```python
from build123d import *

# Parameters (mm, degrees)
F0_W     = 177.8
F0_H     = 101.6
F0_W_2   = 38.1
F0_H_2   = 38.1
F1_DEPTH = 25.4
F2_DEPTH = 0.254


with BuildPart() as f1:
    # F0 (on Front) → F1 (new body)
    with BuildSketch(Plane.XZ):
        with Locations((6.545865, 10.16)):
            Rectangle(F0_W, F0_H)
        with Locations((-62.417315, -15.311638)):
            Rectangle(F0_W_2, F0_H_2, mode=Mode.SUBTRACT)
        with Locations((7.015266, -19.05)):
            Rectangle(F0_W_2, F0_H_2, mode=Mode.SUBTRACT)
        with Locations((66.230962, -19.05)):
            Rectangle(F0_W_2, F0_H_2, mode=Mode.SUBTRACT)
        with Locations((-62.417315, 38.729876)):
            Rectangle(F0_W_2, F0_H_2, mode=Mode.SUBTRACT)
        with Locations((63.931333, 33.843145)):
            Rectangle(F0_W_2, F0_H_2, mode=Mode.SUBTRACT)
        with Locations((7.015266, 38.729876)):
            Rectangle(F0_W_2, F0_H_2, mode=Mode.SUBTRACT)
    extrude(amount=F1_DEPTH)

    # F0 (on Front) → F2 (join)
    with BuildSketch(Plane.XZ):
        with Locations((-62.417315, 38.729876)):
            Rectangle(F0_W_2, F0_H_2)
        with Locations((7.015266, 38.729876)):
            Rectangle(F0_W_2, F0_H_2)
        with Locations((63.931333, 33.843145)):
            Rectangle(F0_W_2, F0_H_2)
        with Locations((66.230962, -19.05)):
            Rectangle(F0_W_2, F0_H_2)
        with Locations((7.015266, -19.05)):
            Rectangle(F0_W_2, F0_H_2)
        with Locations((-62.417315, -15.311638)):
            Rectangle(F0_W_2, F0_H_2)
    extrude(amount=F2_DEPTH)


solid = f1.part
```
Design review of the part built by this model. Coordinates are the model's own, in mm. A direction names the side the tool comes from. Give positions to 0.01 mm unless a question says otherwise; leave off trailing zeros. Order: outer loops, then holes, each group sorted by start corner. A loop starts at its lowest first (then second) coordinate and runs counter-clockwise, first axis right, second up. Notation, with made-up numbers: (83.25, 53.25) -> (132.25, 53.25) arc R14 cw to (132.25, 60.25) -> close; hole circle Ø7 at (-15.5, 38). An arc over 180 degrees is marked (long way). Write each question's results on one line, items separated by ' | '. Start each with the question number.
Q1. Wall thickness on L1, parallel to X at y = -18.25, z = 50.5; L2, parallel to Z at x = -60.5, y = -1.25; L3, parallel to X at y = -0.75, z = -15.5: over which ranges is each line inside the solid? List them lowest first. Write a range as from..to.
Q2. Add section A-A on x = -67.5. Give the boundary of the cut face in (y, z).
Q3. Mouldability with a two-part tool opening along Z and no side actions: class faces 1 (the flat face through (5, -25.4, 11)), 2 (the flat face through (7, -13, -38.1)) as +Z half, -Z half, draft (parallel to the pull), parting line (faces both ways), or undercut.
Q4. Add section B-B on y = -4. Give the boundary of the cut face in (x, z), and give its area (3 significant figures).
Q5. Add section C-C on z = -31. Give the boundary of the cut face in (x, y).
Q6. Machinability: for faces 3 (the flat face through (-43.367, -13, 38)), 4 (the flat face through (95.446, -13, 9)), which of the approach directions +Z, -Z, +X, -X, +Y, -Y give a long, thin tool a straight path to every point of the face, cutting with its end or side? Answer none if there is none.
Q7. For pin 1 (8 mm diameter, centred on x = 6.5, z = -28, fed in from -Y), flat-tipped, find the tip position at first contact; note if it passes through.
Found:
1) L1: x = -82.35..-81.47, -43.37..-12.03, 26.07..44.88, 82.98..95.45 | L2: z = -40.64..-34.36, 3.74..19.68, 57.78..60.96 | L3: x = -82.35..-81.47, -43.37..-12.03, 26.07..47.18, 85.28..95.45
2) outline: (-25.4, -40.64) -> (0, -40.64) -> (0, 60.96) -> (-25.4, 60.96) -> (-25.4, 57.78) -> (-0.25, 57.78) -> (-0.25, 19.68) -> (-25.4, 19.68) -> (-25.4, 3.74) -> (-0.25, 3.74) -> (-0.25, -34.36) -> (-25.4, -34.36) -> close
3) face 1: draft | face 2: undercut
4) outline: (-82.35, -40.64) -> (95.45, -40.64) -> (95.45, 60.96) -> (-82.35, 60.96) -> close; hole (-81.47, -34.36) -> (-43.37, -34.36) -> (-43.37, 3.74) -> (-81.47, 3.74) -> close; hole (-81.47, 19.68) -> (-43.37, 19.68) -> (-43.37, 57.78) -> (-81.47, 57.78) -> close; hole (-12.03, -38.1) -> (26.07, -38.1) -> (26.07, 0) -> (-12.03, 0) -> close; hole (-12.03, 19.68) -> (26.07, 19.68) -> (26.07, 57.78) -> (-12.03, 57.78) -> close; hole (44.88, 14.79) -> (82.98, 14.79) -> (82.98, 52.89) -> (44.88, 52.89) -> close; hole (47.18, -38.1) -> (85.28, -38.1) -> (85.28, 0) -> (47.18, 0) -> close | area: 9,350 mm2
5) outline: (-82.35, -25.4) -> (-81.47, -25.4) -> (-81.47, -0.25) -> (-43.37, -0.25) -> (-43.37, -25.4) -> (-12.03, -25.4) -> (-12.03, -0.25) -> (26.07, -0.25) -> (26.07, -25.4) -> (47.18, -25.4) -> (47.18, -0.25) -> (85.28, -0.25) -> (85.28, -25.4) -> (95.45, -25.4) -> (95.45, 0) -> (-82.35, 0) -> close
6) face 3: -Y | face 4: +Z, -Z, +X, +Y, -Y
7) pin 1: stops at y = -0.25
